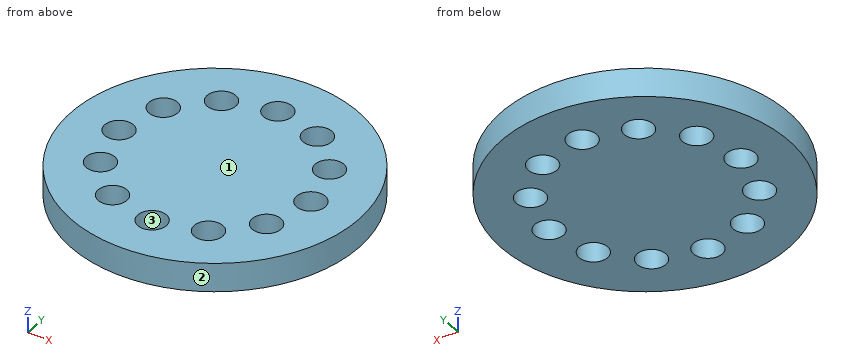
```python
from build123d import *

# Parameters (mm, degrees)
F2_R            = 120
F3_DEPTH        = 24
F4_R            = 12
F5_DEPTH        = 24.001
F5_COPIES_COUNT = 12


# Not quite as in the source:
# - a pattern or mirror of a feature is missing from the dataset's text; its kind, count and spacing are read off the source's solid


with BuildPart() as f3:
    # F2 (on Top) → F3 (new body)
    with BuildSketch(Plane.XY):
        Circle(F2_R)
    extrude(amount=F3_DEPTH)

    # F4 (on face) → F5 (cut, through all)
    with BuildSketch(Plane.XY.offset(24)):
        with Locations((0, 80)):
            Circle(F4_R)
    f5 = extrude(amount=-F5_DEPTH, mode=Mode.SUBTRACT)

    # F5_copies: F5 ×12 about axis
    f5_copies_axis = Axis((0, 0, 0), (0, 0, 1))
    for i in range(1, F5_COPIES_COUNT):
        add(f5.rotate(f5_copies_axis, i * 360 / F5_COPIES_COUNT), mode=Mode.SUBTRACT)


solid = f3.part
```
Part model, mm, in its own coordinate system. Face numbers are marked on the shaded views. Round coordinates to 2 decimals unless told otherwise and drop trailing zeros. Loops run counter-clockwise (first coordinate to the right, second up) from the corner with the lowest first, then second, coordinate; pieces in that order, holes last.
Item 1: Cut at D-D, the plane z = 17.75. State how many separate pieces and enclosed holes the cut face has, then the cut area to 3 significant figures.
Item 2: Cut at C-C, the plane y = -72.5. Give the cut face in (x, z).
Item 3: Mould opens along X. For the marked faces 1, 2 and 3 say: +X half, -X half, draft (parallel to the pull), parting line (faces both ways), or undercut.
Item 4: Drop flat-ended pins along their axis: P1, Ø1.5, axis at y = 51.5, z = 3.5, coming from the -X side; P2, Ø1.5, axis at y = 23.5, z = 14.5, coming from the -X side; P3, Ø4, axis at y = -66, z = 5, coming from the -X side. Give the stop position or say it passes through.
Item 5: Cut at A-A, the plane y = 40. Give the cut face in (x, z).
Item 6: Drill centre lines: line 1 (X direction, y = 31, z = 1.5); line 2 (X direction, y = -74, z = 11.75); line 3 (X direction, y = 31.5, z = 3). Where is each one in solid material? Low to high.
Item 7: Cut at B-B, the plane x = 0. Give the cut face in (y, z).
A:
1. separate pieces: 1
1. enclosed holes: 12
1. area: 39,800 mm2
2. outline: (-95.62, 0) - (-51.56, 0) - (-51.56, 24) - (-95.62, 24) - close; (-28.44, 0) - (-9.37, 0) - (-9.37, 24) - (-28.44, 24) - close; (9.37, 0) - (28.44, 0) - (28.44, 24) - (9.37, 24) - close; (51.56, 0) - (95.62, 0) - (95.62, 24) - (51.56, 24) - close
3. face 1: draft
3. face 2: parting line
3. face 3: undercut
4. P1: stops at x = -108.74
4. P2: stops at x = -117.82
4. P3: stops at x = -101.51
5. outline: (-113.14, 0) - (-81.28, 0) - (-81.28, 24) - (-113.14, 24) - close; (-57.28, 0) - (57.28, 0) - (57.28, 24) - (-57.28, 24) - close; (81.28, 0) - (113.14, 0) - (113.14, 24) - (81.28, 24) - close
6. line 1: x = -115.93 to -77.22, -61.34 to 61.34, 77.22 to 115.93
6. line 2: x = -94.47 to -51.03, -28.97 to -10.39, 10.39 to 28.97, 51.03 to 94.47
6. line 3: x = -115.79 to -77.75, -60.81 to 60.81, 77.75 to 115.79
7. outline: (-120, 0) - (-92, 0) - (-92, 24) - (-120, 24) - close; (-68, 0) - (68, 0) - (68, 24) - (-68, 24) - close; (92, 0) - (120, 0) - (120, 24) - (92, 24) - close
